For this review, take the finished solid that the model builds, in its own axes (mm). Face numbers are marked on the shaded views. A direction names the side the tool comes from. Coordinates: 2 decimals unless noted, no trailing zeros. Loops run counter-clockwise (first coordinate to the right, second up) from the corner with the lowest first, then second, coordinate; pieces in that order, holes last. Notation, with made-up numbers: (-38, 0) -> (-24, 0) arc R9 cw to (-24, 16) -> close; hole circle Ø3 at (-3, 26.25). An arc over 180 degrees is marked (long way). Use a Markdown table: item, result.
from build123d import *

# Parameters (mm, degrees)
BOSS_EXTRUDE1_DEPTH = 2.54
SKETCH2_R           = 2.794
CUT_EXTRUDE1_DEPTH  = 81.372038048
SKETCH3_R           = 3.175
BOSS_EXTRUDE2_DEPTH = 19.05
FILLET1_R           = 5.08


with BuildPart() as part:
    # Sketch1 → Boss-Extrude1 (new body)
    with BuildSketch(Plane.XY):
        with BuildLine():
            Line((16.51, -12.7), (57.15, -12.7))
            ThreePointArc((57.15, -12.7), (60.742102448, -14.187897552), (62.23, -17.78))
            Line((62.23, -17.78), (62.23, -45.72))
            ThreePointArc((62.23, -45.72), (60.742102448, -49.312102448), (57.15, -50.8))
            Line((57.15, -50.8), (16.51, -50.8))
            ThreePointArc((16.51, -50.8), (12.917897552, -49.312102448), (11.43, -45.72))
            Line((11.43, -45.72), (11.43, -17.78))
            ThreePointArc((11.43, -17.78), (12.917897552, -14.187897552), (16.51, -12.7))
        make_face()
    extrude(amount=BOSS_EXTRUDE1_DEPTH)

    # Sketch2 → Cut-Extrude1 (cut, through all)
    with BuildSketch(Plane.XY.offset(2.54)):
        with Locations((24.13, -21.59)):
            Circle(SKETCH2_R)
        with Locations((49.53, -21.59)):
            Circle(SKETCH2_R)
        with Locations((24.13, -41.91)):
            Circle(SKETCH2_R)
        with Locations((49.53, -41.91)):
            Circle(SKETCH2_R)
    extrude(amount=-CUT_EXTRUDE1_DEPTH, mode=Mode.SUBTRACT)

    # Sketch3 → Boss-Extrude2 (add)
    with BuildSketch(Plane.XY.offset(2.54)):
        with Locations(Location((36.83, -31.75, 0), (0, 0, 180))):
            Circle(SKETCH3_R)
    extrude(amount=BOSS_EXTRUDE2_DEPTH)

    # Fillet1
    fillet1_edges = [part.edges().sort_by_distance(p)[0] for p in [
        (40.005, -31.75, 2.54),
    ]]
    fillet(fillet1_edges, radius=FILLET1_R)


solid = part.part
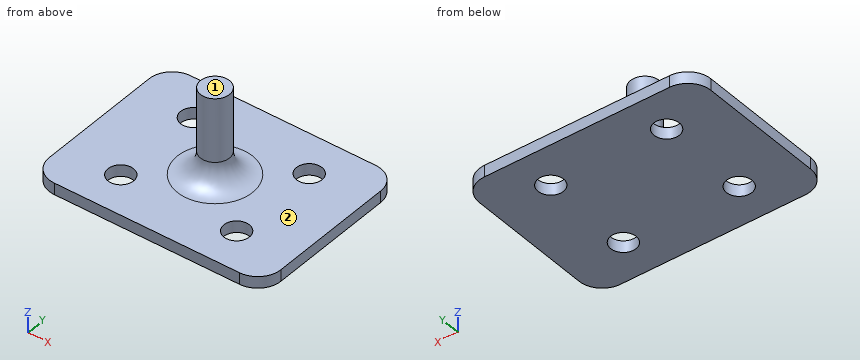
(1) For line 1 along Y through (x, z) = (49.53, 0.65); line 2 along Y through (x, z) = (22.5, 1); line 3 along Z through (x, y) = (55, -44), list the stretches that pass through material, from the lowest coordinate up.
Found:
| item | result |
|---|---|
| line 1 | y = -50.8 to -44.7, -39.12 to -24.38, -18.8 to -12.7 |
| line 2 | y = -50.8 to -44.18, -39.64 to -23.86, -19.32 to -12.7 |
| line 3 | z = 0 to 2.54 |
(2) For pin 1 Ø6.5 at (x, y) = (24.13, -41.91) entering from +Z; pin 2 Ø19 at (x, y) = (48, -23) entering from +Z; pin 3 Ø1 at (x, z) = (31, 5) entering from -Y, all flat-tipped, find the tip position at first contact; note any pin that passes through.
Found:
| item | result |
|---|---|
| pin 1 | stops at z = 2.54 |
| pin 2 | stops at z = 4 |
| pin 3 | passes through |
(3) Take a section at B-B on x = 24.13. Write out the cut boundary in (y, z).
Found:
| item | result |
|---|---|
| outline | (-50.8, 0) -> (-44.7, 0) -> (-44.7, 2.54) -> (-50.8, 2.54) -> close; (-39.12, 0) -> (-24.38, 0) -> (-24.38, 2.54) -> (-39.12, 2.54) -> close; (-18.8, 0) -> (-12.7, 0) -> (-12.7, 2.54) -> (-18.8, 2.54) -> close |
(4) For the marked faces 1 and 2, list the 3-axis set-ups (+Z, -Z, +X, -X, +Y, -Y) from which the entire face can be reached by the end or side of a thin tool; tool diameter is ignored.
Found:
| item | result |
|---|---|
| face 1 | +Z, +X, -X, +Y, -Y |
| face 2 | +Z |
(5) Take a section at A-A on y = -21.59. Write out the cut boundary in (x, z), plus the area to 3 significant figures.
Found:
| item | result |
|---|---|
| outline | (11.43, 0) -> (21.34, 0) -> (21.34, 2.54) -> (11.43, 2.54) -> close; (26.92, 0) -> (46.74, 0) -> (46.74, 2.54) -> (26.92, 2.54) -> close; (52.32, 0) -> (62.23, 0) -> (62.23, 2.54) -> (52.32, 2.54) -> close |
| area | 101 mm^2 |
(6) Take a section at D-D on z = 18.25. Write out the cut boundary in (x, y) (3 decimals).
Found:
| item | result |
|---|---|
| outline | circle Ø6.35 at (36.83, -31.75) |
(7) Take a section at C-C on x = 36.83. Write out the cut boundary in (y, z) (3 decimals), plus the area to 3 significant figures.
Found:
| item | result |
|---|---|
| outline | (-50.8, 0) -> (-12.7, 0) -> (-12.7, 2.54) -> (-23.495, 2.54) arc R5.08 cw to (-28.575, 7.62) -> (-28.575, 21.59) -> (-34.925, 21.59) -> (-34.925, 7.62) arc R5.08 cw to (-40.005, 2.54) -> (-50.8, 2.54) -> close |
| area | 229 mm^2 |
